from build123d import *

# Parameters (mm, degrees)
BOSS_EXTRUDE1_DEPTH                            = 4
SKETCH2_R                                      = 2.25
CUT_EXTRUDE1_DEPTH                             = 46
SKETCH2_3_R                                    = 2.15
BOSS_EXTRUDE2_DEPTH                            = 8
BOSS_EXTRUDE4_DEPTH                            = 8
SKETCH6_W                                      = 11.5
SKETCH6_H                                      = 18.413961031
CUT_EXTRUDE2_DEPTH                             = 47.400431032
SKETCH12_W                                     = 8
SKETCH12_H                                     = 13.1
CUT_EXTRUDE3_DEPTH                             = 40.286161686
CBORE_FOR_6_SOCKET_HEAD_CAP_SCREW1_D           = 3.6576
CBORE_FOR_6_SOCKET_HEAD_CAP_SCREW1_CBORE_D     = 7
CBORE_FOR_6_SOCKET_HEAD_CAP_SCREW1_CBORE_DEPTH = 3.5052
SKETCH13_W                                     = 11.5
SKETCH13_H                                     = 16.586038969
CUT_EXTRUDE4_DEPTH                             = 5
CUT_EXTRUDE5_START                             = -1.5
SKETCH14_R                                     = 2.15
CUT_EXTRUDE5_DEPTH                             = 1.5


with BuildPart() as part:
    # Sketch1 → Boss-Extrude1 (new body)
    with BuildSketch(Plane.XY):
        with BuildLine():
            Line((18, 0), (28, 10))
            Line((28, 10), (28, 33))
            ThreePointArc((28, 33), (27.414213562, 34.414213562), (26, 35))
            Line((26, 35), (0, 35))
            Line((0, 35), (0, 0))
            Line((0, 0), (18, 0))
        make_face()
    extrude(amount=BOSS_EXTRUDE1_DEPTH)

    # Sketch2 → Cut-Extrude1 (cut, through all)
    with BuildSketch(Plane(origin=(0, 0, 0), x_dir=(-1, 0, 0), z_dir=(0, 0, -1))):
        with Locations((-23.5, 11.863961031)):
            Circle(SKETCH2_R)
    extrude(amount=-CUT_EXTRUDE1_DEPTH, mode=Mode.SUBTRACT)

    # Sketch2<3> → Boss-Extrude2 (add)
    with BuildSketch(Plane(origin=(0, 0, 0), x_dir=(-1, 0, 0), z_dir=(0, 0, -1))):
        with Locations(Location((-23.5, 29.863961031, 0), (0, 0, 180))):
            Circle(SKETCH2_3_R)
    extrude(amount=BOSS_EXTRUDE2_DEPTH)

    # Sketch2<5> → Boss-Extrude4 (add)
    with BuildSketch(Plane(origin=(0, 0, 0), x_dir=(-1, 0, 0), z_dir=(0, 0, -1))):
        with BuildLine():
            ThreePointArc((-26.5, 18.792344681), (-23.077745882, 19.402143932), (-19.745003329, 18.413961031))
            Line((-19.745003329, 18.413961031), (-15.95, 18.413961031))
            Line((-15.95, 18.413961031), (-15.95, 5.313961031))
            Line((-15.95, 5.313961031), (-19.725, 5.313961031))
            ThreePointArc((-19.725, 5.313961031), (-20.25595921, 5.035394245), (-20.807324798, 4.799782009))
            ThreePointArc((-20.807324798, 4.799782009), (-21.429052247, 4.074422526), (-21.15825613, 3.15825613))
            Line((-21.15825613, 3.15825613), (-18, 0))
            Line((-18, 0), (0, 0))
            Line((0, 0), (0, 35))
            Line((0, 35), (-16, 35))
            Line((-16, 35), (-16, 29.863961031))
            ThreePointArc((-16, 29.863961031), (-19.392080819, 23.589010832), (-26.5, 22.990097488))
            Line((-26.5, 22.990097488), (-26.5, 18.792344681))
        make_face()
    extrude(amount=BOSS_EXTRUDE4_DEPTH)

    # Sketch6 → Cut-Extrude2 (cut, through all)
    with BuildSketch(Plane(origin=(0, 0, -8), x_dir=(-1, 0, 0), z_dir=(0, 0, -1))):
        with Locations((-5.75, 9.206980515)):
            Rectangle(SKETCH6_W, SKETCH6_H)
    extrude(amount=-CUT_EXTRUDE2_DEPTH, mode=Mode.SUBTRACT)

    # Sketch12 → Cut-Extrude3 (cut, through all)
    with BuildSketch(Plane(origin=(15.95, 0, 0), x_dir=(0, 0, -1), z_dir=(1, 0, 0))):
        with Locations((4, 11.863961031)):
            Rectangle(SKETCH12_W, SKETCH12_H)
    extrude(amount=-CUT_EXTRUDE3_DEPTH, mode=Mode.SUBTRACT)

    # CBORE for #6 Socket Head Cap Screw1 (through all)
    with Locations(Plane.XY.offset(4)):
        with Locations((6.35, 26)):
            CounterBoreHole(CBORE_FOR_6_SOCKET_HEAD_CAP_SCREW1_D / 2, CBORE_FOR_6_SOCKET_HEAD_CAP_SCREW1_CBORE_D / 2, CBORE_FOR_6_SOCKET_HEAD_CAP_SCREW1_CBORE_DEPTH)

    # Sketch13 → Cut-Extrude4 (cut)
    with BuildSketch(Plane(origin=(0, 0, -8), x_dir=(-1, 0, 0), z_dir=(0, 0, -1))):
        with Locations((-5.75, 26.706980515)):
            Rectangle(SKETCH13_W, SKETCH13_H)
    extrude(amount=-CUT_EXTRUDE4_DEPTH, mode=Mode.SUBTRACT)

    # Sketch14 → Cut-Extrude5 (cut)
    with BuildSketch(Plane(origin=(0, 0, -8), x_dir=(-1, 0, 0), z_dir=(0, 0, -1)).offset(CUT_EXTRUDE5_START)):
        with Locations(Location((-23.5, 29.863961031, 0), (0, 0, 180))):
            Circle(SKETCH14_R)
    extrude(amount=CUT_EXTRUDE5_DEPTH, mode=Mode.SUBTRACT)


solid = part.part
The model under review builds one solid part; all positions refer to its coordinate system, in mm. A direction names the side the tool comes from. Give positions to 0.01 mm unless a question says otherwise; leave off trailing zeros. Write each loop counter-clockwise with the first axis right and the second up, starting at its lowest first coordinate (ties: lowest second). Pieces come first, ordered by that corner, then holes. Notation, with made-up numbers: M 21.5,1 L 40.5,1 A17 cw 40.5,31 Z; hole C 82.5,-28.5 d7. An arc over 180 degrees is marked long. One line per question, with ' | ' between items. Start each with the question number.
Item 1: Wall thickness on line 1 (Y direction, x = 6.35, z = 2.1); line 2 (Y direction, x = 6.35, z = -0.6); line 3 (Z direction, x = 17.5, y = 28): over which ranges is each line inside the solid? List them lowest first. Write a range as from..to.
Item 2: We need section D-D on y = 20.5. Write out the cut boundary in (x, z), plus the area to 4 significant figures.
Item 3: For pin 1 (6 mm diameter, centred on x = 7, y = 30, fed in from -Z); pin 2 (4.5 mm diameter, centred on y = 21, z = -2, fed in from +X); pin 3 (4.5 mm diameter, centred on x = 23, y = 30.5, fed in from -Z); pin 4 (4 mm diameter, centred on y = 29.5, z = -5.5, fed in from -X), all flat-tipped, find the tip position at first contact; note any pin that passes through.
Item 4: For faces 5 (the cylindrical face through (20.25, 5.04, -3.94)), 6 (the flat face through (6, 29, -3)), 7 (the flat face through (26.5, 21, -4)), 8 (the cylindrical face through (23.03, 31.96, -3.2)), 9 (the flat face through (16, 5.314, -4)), list the 3-axis set-ups (+Z, -Z, +X, -X, +Y, -Y) from which the entire face can be reached by the end or side of a thin tool; tool diameter is ignored.
Item 5: We need section B-B on z = -5.75. Write out the cut boundary in (x, y) (3 decimals).
Item 6: We need section A-A on x = 6.35. Write out the cut boundary in (y, z), plus the area to 3 significant figures.
Item 7: We need section C-C on x = 12.5. Write out the cut boundary in (y, z).
Item 8: Draft analysis for pull direction Y (two halves, no side actions). For faces 1 (the flat face through (22, 4, 1)), 2 (the flat face through (13, 35, 1)), 3 (the cylindrical face through (23.127, 19.405, -3.944)), 4 (the flat face through (17, 3, -8)), state which applies: released by +Y, released by -Y, zero draft, split by the parting line, or undercut.
Results found:
1) line 1: y = 18.41..22.5, 29.5..35 | line 2: y = 18.41..24.17, 27.83..35 | line 3: z = 0..4
2) outline: M 0,-3 L 11.5,-3 L 11.5,-8 L 26.5,-8 L 26.5,0 L 28,0 L 28,4 L 0,4 Z | area: 266.5 mm2
3) pin 1: stops at z = -3 | pin 2: stops at x = 28 | pin 3: stops at z = -6.5 | pin 4: stops at x = 11.5
4) face 5: -Z, +X | face 6: -Z, -X, +Y, -Y | face 7: -Z, +X, +Y, -Y | face 8: -Z | face 9: -Z, +X, -X
5) outline: M 11.5,0 L 18,0 L 21.158,3.158 A1 ccw 20.807,4.8 A7.56 cw 19.725,5.314 L 11.5,5.314 Z; M 11.5,18.414 L 19.745,18.414 A7.55 cw 26.5,18.792 L 26.5,22.99 A7.5 cw 16,29.864 L 16,35 L 11.5,35 Z; C 23.5,29.864 d4.3
6) outline: M 18.41,-3 L 24.17,-3 L 24.17,0.49 L 22.5,0.49 L 22.5,4 L 18.41,4 Z; M 27.83,-3 L 35,-3 L 35,4 L 29.5,4 L 29.5,0.49 L 27.83,0.49 Z | area: 78.8 mm2
7) outline: M 0,-8 L 5.31,-8 L 5.31,0 L 18.41,0 L 18.41,-8 L 35,-8 L 35,4 L 0,4 Z
8) face 1: released by -Y | face 2: released by +Y | face 3: undercut | face 4: zero draft
